Source: CAD feature listing. Evaluate the final solid. Frame: model axes, mm. A direction names the side the tool comes from. Coordinates: 2 decimals unless noted, no trailing zeros. Order: outer loops, then holes, each group sorted by start corner. A loop starts at its lowest first (then second) coordinate and runs counter-clockwise, first axis right, second up. Notation, with made-up numbers: (22, 14) - (39, 14) arc R22 cw to (39, 21) - close; hole circle Ø11 at (-2, 9). An arc over 180 degrees is marked (long way). One line per question, with ' | ' between items. Start each with the question number.
(1) Draft query along Y for faces 4 (the flat face through (-240, 130, -171)), 5 (the flat face through (-215, 2, 0)), 6 (the flat face through (-1, -175, 1)). Return one class per face: +Y half, -Y half, draft (parallel to the pull), parting line (faces both ways), or undercut.
(2) Section D-D (z = -80). Return the cut outline in (x, y).
(3) Section B-B (x = -209.5). Return the cut outline in (y, z), then the cut area to 4 significant figures.
(4) Contact query for flat-ended pins moving along their axis: P1, Ø2, axis at x = 33.5, y = 107, coming from the -Z side; P2, Ø6, axis at x = 57, y = 113.5, coming from the +Z side. Output: stop coordinate, or through.
(5) Section C-C (y = 136). Return the cut outline in (x, z), then the cut area to 3 significant figures.
(6) Line query: line 1 along Y through (x, z) = (0, 278); line 2 along Y through (x, z) = (-203.5, -86); line 3 along Z through (x, y) = (111.5, 30). Output: solid intervals per line, ascending.
(7) Section A-A (z = -429). Return the cut outline in (x, y), then the cut area to 3 significant figures.
(8) Access query for faces 1 (the cylindrical face through (-29.6, -22.7, 223.2)), 2 (the flat face through (-215, -125, -333)), 3 (the flat face through (190, 150, -414)). Directions: +Z, -Z, +X, -X, +Y, -Y. A direction counts if a zero-diameter tool reaches every point of the face in a straight line with its end or side. Return the directions, or none.
from build123d import *

# Parameters (mm, degrees)
F0_W      = 480
F0_H      = 350
F1_DEPTH  = 100
F2_W      = 50
F2_H      = 50
F3_DEPTH  = 675
F4_W      = 50
F4_H      = 50
F5_DEPTH  = 675
F6_W      = 50
F6_H      = 50
F7_DEPTH  = 675
F8_W      = 50
F8_H      = 50
F9_DEPTH  = 675
F10_R     = 50
F10_R_2   = 37.3037381585
F11_DEPTH = 250
F14_W     = 430
F14_H     = 139.1179516912
F15_DEPTH = 160
F16_DEPTH = 209
F17_W     = 49.8938559854
F17_H     = 160
F18_DEPTH = 430


# Not quite as in the source:
# - a feature names something its author has since deleted; it is built from what else it names
# - the program builds the solid bodies; features that only make, move or delete a surface that nothing else refers to are left out


with BuildPart() as f1:
    # F0 (on Top) → F1 (new body)
    with BuildSketch(Plane.XY):
        Rectangle(F0_W, F0_H)
    extrude(amount=F1_DEPTH)

    # F2 (on face) → F3 (join)
    with BuildSketch(Plane(origin=(0, 0, 0), x_dir=(1, 0, 0), z_dir=(0, 0, -1))):
        with Locations((215, 150)):
            Rectangle(F2_W, F2_H)
    extrude(amount=F3_DEPTH)

    # F4 (on face) → F5 (join)
    with BuildSketch(Plane(origin=(0, 0, 0), x_dir=(1, 0, 0), z_dir=(0, 0, -1))):
        with Locations((215, -150)):
            Rectangle(F4_W, F4_H)
    extrude(amount=F5_DEPTH)

    # F6 (on face) → F7 (join)
    with BuildSketch(Plane(origin=(0, 0, 0), x_dir=(1, 0, 0), z_dir=(0, 0, -1))):
        with Locations((-215, -150)):
            Rectangle(F6_W, F6_H)
    extrude(amount=F7_DEPTH)

    # F8 (on face) → F9 (join)
    with BuildSketch(Plane(origin=(0, 0, 0), x_dir=(1, 0, 0), z_dir=(0, 0, -1))):
        with Locations((-215, 150)):
            Rectangle(F8_W, F8_H)
    extrude(amount=F9_DEPTH)

    # F10 (on face) → F11 (join)
    with BuildSketch(Plane.XY.offset(100)):
        Circle(F10_R)
        Circle(F10_R_2, mode=Mode.SUBTRACT)
    extrude(amount=F11_DEPTH)

    # F14 (on face) → F15 (join)
    with BuildSketch(Plane(origin=(0, 0, 0), x_dir=(1, 0, 0), z_dir=(0, 0, -1))):
        with Locations((25, -105.4410241544)):
            Rectangle(F14_W, F14_H)
    extrude(amount=F15_DEPTH)

    # F16 (add): a face of the model
    f16_faces = [f1.faces().sort_by_distance(p)[0] for p in [
        (25, 35.8820483088, -80),
    ]]
    extrude(f16_faces, amount=F16_DEPTH)

    # F17 (on face) → F18 (join)
    with BuildSketch(Plane(origin=(-190, 0, 0), x_dir=(0, -1, 0), z_dir=(-1, 0, 0))):
        with Locations((-149.9469279927, -80)):
            Rectangle(F17_W, F17_H)
    extrude(amount=-F18_DEPTH)


solid = f1.part
Response values:
1) face 4: draft | face 5: undercut | face 6: -Y half
2) outline: (-240, -175) - (-190, -175) - (-190, -173.12) - (190, -173.12) - (190, -175) - (240, -175) - (240, 175) - (-240, 175) - (-240, 125) - (-190, 125) - (-190, -125) - (-240, -125) - close
3) outline: (-175, -675) - (-125, -675) - (-125, 0) - (125, 0) - (125, -675) - (175, -675) - (175, 100) - (-175, 100) - close | area: 102,500 mm²
4) P1: stops at z = -160 | P2: stops at z = 100
5) outline: (-240, -675) - (-190, -675) - (-190, -160) - (190, -160) - (190, -675) - (240, -675) - (240, 100) - (-240, 100) - close | area: 176,000 mm²
6) line 1: y = -50 to -37.3, 37.3 to 50 | line 2: y = -175 to -125, 125 to 175 | line 3: z = -160 to 100
7) outline: (-240, -175) - (-190, -175) - (-190, -125) - (-240, -125) - close; (-240, 125) - (-190, 125) - (-190, 175) - (-240, 175) - close; (190, -175) - (240, -175) - (240, -125) - (190, -125) - close; (190, 125) - (240, 125) - (240, 175) - (190, 175) - close | area: 10,000 mm²
8) face 1: +Z | face 2: -Z, -X | face 3: -Z, +Y, -Y
